Check sheet for the modelled part. Datum: model origin and axes. Units: mm. A direction names the side the tool comes from. Give positions to 0.01 mm unless a question says otherwise; leave off trailing zeros. Order: outer loops, then holes, each group sorted by start corner. A loop starts at its lowest first (then second) coordinate and runs counter-clockwise, first axis right, second up. Notation, with made-up numbers: M 40.5,81 L 56.5,81 A21 ccw 56.5,90 Z; hole C 39.5,87 d4. An arc over 180 degrees is marked long. Return JSON: item names as keys, results as strings. Group by question number.
from build123d import *

# Parameters (mm, degrees)
SKETCH1_R           = 15
BOSS_EXTRUDE1_DEPTH = 25
SKETCH4_R           = 14.25
SKETCH4_R_2         = 13.5
CUT_EXTRUDE2_DEPTH  = 3
SKETCH5_R           = 2.5
CUT_EXTRUDE3_DEPTH  = 22
SKETCH6_R           = 2.5
CUT_EXTRUDE4_DEPTH  = 10


with BuildPart() as part:
    # Sketch1 → Boss-Extrude1 (new body)
    with BuildSketch(Plane(origin=(0, 0, 0), x_dir=(1, 0, 0), z_dir=(0, 1, 0))):
        with Locations(Location((0, 0, 0), (0, 0, 270))):
            Circle(SKETCH1_R)
    extrude(amount=BOSS_EXTRUDE1_DEPTH)

    # Sketch4 → Cut-Extrude2 (cut)
    with BuildSketch(Plane(origin=(0, 25, 0), x_dir=(1, 0, 0), z_dir=(0, 1, 0))):
        with Locations(Location((0, 0, 0), (0, 0, 270))):
            Circle(SKETCH4_R)
        with Locations(Location((0, 0, 0), (0, 0, 270))):
            Circle(SKETCH4_R_2, mode=Mode.SUBTRACT)
    extrude(amount=-CUT_EXTRUDE2_DEPTH, mode=Mode.SUBTRACT)

    # Sketch5 → Cut-Extrude3 (cut)
    with BuildSketch(Plane(origin=(0, 25, 0), x_dir=(1, 0, 0), z_dir=(0, 1, 0))):
        with Locations(Location((0, 7, 0), (0, 0, 270))):
            Circle(SKETCH5_R)
        with Locations(Location((6.062177826, 3.5, 0), (0, 0, 270))):
            Circle(SKETCH5_R)
        with Locations(Location((6.062177826, -3.5, 0), (0, 0, 270))):
            Circle(SKETCH5_R)
        with Locations(Location((0, -7, 0), (0, 0, 270))):
            Circle(SKETCH5_R)
        with Locations(Location((-6.062177826, -3.5, 0), (0, 0, 270))):
            Circle(SKETCH5_R)
        with Locations(Location((-6.062177826, 3.5, 0), (0, 0, 270))):
            Circle(SKETCH5_R)
    extrude(amount=-CUT_EXTRUDE3_DEPTH, mode=Mode.SUBTRACT)

    # Sketch6 → Cut-Extrude4 (cut)
    with BuildSketch(Plane.XZ):
        with Locations(Location((0, 0, 0), (0, 0, 270))):
            Circle(SKETCH6_R)
    extrude(amount=-CUT_EXTRUDE4_DEPTH, mode=Mode.SUBTRACT)


solid = part.part
1) Sectioned sample at C-C on z = -3.75. Record the boundary of the cut face in (x, y), then the cut area to 3 significant figures.
2) Release check for a two-part mould opening along X. For faces 1 (the face through (0.66, 12.325, -14.985)), 2 (the face through (0, 3, 7)), 3 (the face through (0, 0, 3)) record: released by +X, released by -X, zero draft, split by the parting line, or undercut.
3) Sectioned sample at A-A on x = 0. Record the boundary of the cut face in (y, z).
4) Depth check by flat-ended pin: P1, Ø1.5, axis at x = -0.5, z = 0, coming from the -Y side; P2, Ø1.5, axis at x = 7, z = 4, coming from the +Y side; P3, Ø2, axis at x = 4, y = 20.5, coming from the -Z side. Enter the tip coordinate at first touch or a pass-through.
5) Material ranges on line 1 along X through (y, z) = (12.75, -2.5); line 2 along X through (y, z) = (17, -3.5); line 3 along Z through (x, y) = (-9.75, 23.75), recorded low to high.
6) Sectioned sample at B-B on y = 11.75. Record the boundary of the cut face in (x, z), then the cut area to 3 significant figures.
7) Sectioned sample at D-D on y = 8. Record the boundary of the cut face in (x, z).
8) Tool access check on faces 4 (the face through (-12, 25, 8)), 5 (the face through (3.844, 14.154, 4.654)). Record the directions out of +Z, -Z, +X, -X, +Y, -Y that give a thin tool (end or side, any length) a straight path to the whole face; none if there is none.
Reply:
{
 "1": {"outline": "M -14.52,0 L 14.52,0 L 14.52,25 L 13.75,25 L 13.75,22 L 12.97,22 L 12.97,25 L 8.55,25 L 8.55,3 L 3.57,3 L 3.57,25 L -3.57,25 L -3.57,3 L -8.55,3 L -8.55,25 L -12.97,25 L -12.97,22 L -13.75,22 L -13.75,25 L -14.52,25 Z", "area": "503 mm^2"},
 "2": {"face 1": "split by the parting line", "face 2": "undercut", "face 3": "zero draft"},
 "3": {"outline": "M 0,-15 L 25,-15 L 25,-14.25 L 22,-14.25 L 22,-13.5 L 25,-13.5 L 25,-9.5 L 3,-9.5 L 3,-4.5 L 25,-4.5 L 25,4.5 L 3,4.5 L 3,9.5 L 25,9.5 L 25,13.5 L 22,13.5 L 22,14.25 L 25,14.25 L 25,15 L 0,15 L 0,2.5 L 10,2.5 L 10,-2.5 L 0,-2.5 Z"},
 "4": {"P1": "y = 10", "P2": "y = 3", "P3": "z = -14.7"},
 "5": {"line 1": "-14.79 to -8.35, -3.77 to 3.77, 8.35 to 14.79", "line 2": "-14.59 to -8.56, -3.56 to 3.56, 8.56 to 14.59", "line 3": "-11.4 to -10.39, -9.34 to 9.34, 10.39 to 11.4"},
 "6": {"outline": "C 0,0 d30; hole C -6.06,-3.5 d5; hole C -6.06,3.5 d5; hole C 0,-7 d5; hole C 0,7 d5; hole C 6.06,-3.5 d5; hole C 6.06,3.5 d5", "area": "589 mm^2"},
 "7": {"outline": "C 0,0 d30; hole C -6.06,-3.5 d5; hole C -6.06,3.5 d5; hole C 0,-7 d5; hole C 0,0 d5; hole C 0,7 d5; hole C 6.06,-3.5 d5; hole C 6.06,3.5 d5"},
 "8": {"face 4": "+Z, -Z, +X, -X, +Y", "face 5": "+Y"}
}
